Input: part model. Units: mm. Frame: model coordinates. A direction names the side the tool comes from. Give positions to 0.01 mm unless a question says otherwise; leave off trailing zeros. Loops run counter-clockwise (first coordinate to the right, second up) from the corner with the lowest first, then second, coordinate; pieces in that order, holes last. Notation, with made-up numbers: M 71.25,-22.5 L 102.25,-22.5 A20 ccw 102.25,-5.5 Z; hole C -21.5,46 d9. An arc over 180 degrees is marked long. Use CSV: the item, a comma, the result in double quotes. Start each with the question number.
Q1. Pin query (flat end, axial travel): pin 1 (20.5 mm diameter, centred on x = 49.5, z = 49.5, fed in from -Y); pin 2 (14.5 mm diameter, centred on x = -49.5, z = 49.5, fed in from -Y); pin 3 (7 mm diameter, centred on x = -45.96, z = 45.96, fed in from -Y). Return the tip coordinate at first contact, or that it passes through.
Q2. Section D-D, the plane y = -36. Output: boundary loops of the cut face in (x, z), plus the area to 3 significant figures.
Q3. Section C-C, the plane x = 69.5. Output: boundary loops of the cut face in (y, z).
Q4. Pull-direction query (X, two-part tool) for faces 6 (the cylindrical face through (-34.05, 53.52, -41.21)), 7 (the flat face through (88.5, -1, 1)), 8 (the flat face through (-21, 56.475, 29)); classes: released by +X, released by -X, zero draft, split by the parting line, or undercut.
Q5. Section A-A, the plane x = 0. Output: boundary loops of the cut face in (y, z), plus the area to 3 significant figures.
Q6. Section B-B, the plane z = 0. Output: boundary loops of the cut face in (x, y), plus the area to 3 significant figures.
Q7. Reachability of faces 1 (the flat face through (-0.413, -54.646, 92.014)), 2 (the flat face through (-41, -56.475, -40)), 3 (the cylindrical face through (52.945, -53.517, 57.811)), 4 (the flat face through (-19.5, 50.475, 29.4)), 5 (the cylindrical face through (-5.48, 53.52, -44.86)) from +Z, -Z, +X, -X, +Y, -Y: full face, straight path, thin tool, end or side. Return the list, or none.
Q8. Material intervals for line 1 along X through (y, z) = (22, 34); line 2 along Y through (x, z) = (65.5, -42); line 3 along Y through (x, z) = (-18, -38), sorted ascending.
from build123d import *

# Parameters (mm, degrees)
SKETCH1_W           = 177
SKETCH1_H           = 112.94900091
SKETCH1_W_2         = 165
SKETCH1_H_2         = 100.94900091
EXTRUDE_THIN1_DEPTH = 92.5
CUT_EXTRUDE1_REACH  = 172.722
SKETCH2_R           = 35
SKETCH2_R_2         = 6
SKETCH3_R           = 50
SKETCH3_R_2         = 9
CUT_EXTRUDE2_DEPTH  = 10
CUT_EXTRUDE3_DEPTH  = 208.544258417
CIRPATTERN1_COUNT   = 4
SKETCH5_R           = 9
CUT_EXTRUDE4_DEPTH  = 10


with BuildPart() as part:
    # Sketch1 → Extrude-Thin1 (new, symmetric)
    with BuildSketch(Plane.XY):
        Rectangle(SKETCH1_W, SKETCH1_H)
        Rectangle(SKETCH1_W_2, SKETCH1_H_2, mode=Mode.SUBTRACT)
    extrude(amount=EXTRUDE_THIN1_DEPTH, both=True)

    # Sketch2 → Cut-Extrude1 (cut, up to next)
    with BuildSketch(Plane(origin=(0, 56.474500455, 0), x_dir=(1, 0, 0), z_dir=(0, 1, 0)), mode=Mode.PRIVATE) as cut_extrude1_sk1:
        with Locations(Location((0, 0, 0), (0, 0, 270))):
            Circle(SKETCH2_R)
    cut_extrude1_tool1 = extrude(cut_extrude1_sk1.sketch, amount=-CUT_EXTRUDE1_REACH, mode=Mode.PRIVATE) & part.part
    # Sketch2 → Cut-Extrude1 (cut, up to next)
    with BuildSketch(Plane(origin=(0, 56.474500455, 0), x_dir=(1, 0, 0), z_dir=(0, 1, 0)), mode=Mode.PRIVATE) as cut_extrude1_sk2:
        with Locations(Location((-35.355339059, -35.355339059, 0), (0, 0, 270))):
            Circle(SKETCH2_R_2)
    cut_extrude1_tool2 = extrude(cut_extrude1_sk2.sketch, amount=-CUT_EXTRUDE1_REACH, mode=Mode.PRIVATE) & part.part
    # Sketch2 → Cut-Extrude1 (cut, up to next)
    with BuildSketch(Plane(origin=(0, 56.474500455, 0), x_dir=(1, 0, 0), z_dir=(0, 1, 0)), mode=Mode.PRIVATE) as cut_extrude1_sk3:
        with Locations(Location((-45.961940777, -45.961940777, 0), (0, 0, 270))):
            Circle(SKETCH2_R_2)
    cut_extrude1_tool3 = extrude(cut_extrude1_sk3.sketch, amount=-CUT_EXTRUDE1_REACH, mode=Mode.PRIVATE) & part.part
    cut_extrude1_1 = cut_extrude1_tool1.solids().sort_by_distance((0, 56.4745, 0))[0]
    add(cut_extrude1_1, mode=Mode.SUBTRACT)
    cut_extrude1_2 = cut_extrude1_tool2.solids().sort_by_distance((-35.355339, 56.4745, 35.355339))[0]
    add(cut_extrude1_2, mode=Mode.SUBTRACT)
    cut_extrude1_3 = cut_extrude1_tool3.solids().sort_by_distance((-45.961941, 56.4745, 45.961941))[0]
    add(cut_extrude1_3, mode=Mode.SUBTRACT)
    cut_extrude1 = cut_extrude1_1 + cut_extrude1_2 + cut_extrude1_3  # Cut-Extrude1 as one shape, for the pattern or mirror that repeats it

    # Sketch3 → Cut-Extrude2 (cut)
    with BuildSketch(Plane.XZ.offset(56.474500455)):
        with Locations(Location((0, 0, 0), (0, 0, 270))):
            Circle(SKETCH3_R)
        with Locations(Location((-49.497474683, -49.497474683, 0), (0, 0, 270))):
            Circle(SKETCH3_R_2)
    cut_extrude2 = extrude(amount=-CUT_EXTRUDE2_DEPTH, mode=Mode.SUBTRACT)

    # Sketch4 → Cut-Extrude3 (cut, through all)
    with BuildSketch(Plane.ZY.offset(88.5)):
        Polygon((-92.5, -56.474500455), (-62.5, 56.474500455), (-92.5, 56.474500455), align=None)
    cut_extrude3 = extrude(amount=-CUT_EXTRUDE3_DEPTH, mode=Mode.SUBTRACT)

    # Mirror1: Cut-Extrude3 across plane
    add(cut_extrude3.mirror(Plane.XY), mode=Mode.SUBTRACT)

    # CirPattern1: Cut-Extrude1, Cut-Extrude2 ×4 about axis
    cirpattern1_axis = Axis((0, 0, 0), (0, 1, 0))
    add([cut_extrude1.rotate(cirpattern1_axis, i * 360 / CIRPATTERN1_COUNT) for i in range(1, CIRPATTERN1_COUNT)], mode=Mode.SUBTRACT)
    add([cut_extrude2.rotate(cirpattern1_axis, i * 360 / CIRPATTERN1_COUNT) for i in range(1, CIRPATTERN1_COUNT)], mode=Mode.SUBTRACT)

    # Sketch5 → Cut-Extrude4 (cut)
    with BuildSketch(Plane(origin=(0, 56.474500455, 0), x_dir=(1, 0, 0), z_dir=(0, 1, 0))):
        with Locations(Location((0, -52, 0), (0, 0, 270))):
            Circle(SKETCH5_R)
    cut_extrude4 = extrude(amount=-CUT_EXTRUDE4_DEPTH, mode=Mode.SUBTRACT)

    # Mirror2: Cut-Extrude4 across plane
    add(cut_extrude4.mirror(Plane.XY), mode=Mode.SUBTRACT)


solid = part.part
A:
1,pin 1,"y = -56.47"
1,pin 2,"y = 50.47"
1,pin 3,"through"
2,outline,"M -88.5,-87.06 L -82.5,-87.06 L -82.5,87.06 L -88.5,87.06 Z; M 82.5,-87.06 L 88.5,-87.06 L 88.5,87.06 L 82.5,87.06 Z"
2,area,"2,090 mm^2"
3,outline,"M -56.47,-92.5 L -50.47,-90.91 L -50.47,90.91 L -56.47,92.5 Z; M 50.47,-64.09 L 56.47,-62.5 L 56.47,62.5 L 50.47,64.09 Z"
4,face 6,"undercut"
4,face 7,"released by +X"
4,face 8,"zero draft"
5,outline,"M -56.47,-92.5 L -50.47,-90.91 L -50.47,-50 L -56.47,-50 Z; M -56.47,50 L -50.47,50 L -50.47,90.91 L -56.47,92.5 Z; M 50.47,-64.09 L 56.47,-62.5 L 56.47,-61 L 50.47,-61 Z; M 50.47,-43 L 56.47,-43 L 56.47,-35 L 50.47,-35 Z; M 50.47,35 L 56.47,35 L 56.47,43 L 50.47,43 Z; M 50.47,61 L 56.47,61 L 56.47,62.5 L 50.47,64.09 Z"
5,area,"624 mm^2"
6,outline,"M -88.5,-56.47 L -50,-56.47 L -50,-50.47 L -82.5,-50.47 L -82.5,50.47 L -35,50.47 L -35,56.47 L -88.5,56.47 Z; M 35,50.47 L 82.5,50.47 L 82.5,-50.47 L 50,-50.47 L 50,-56.47 L 88.5,-56.47 L 88.5,56.47 L 35,56.47 Z"
6,area,"2,320 mm^2"
7,face 1,"+Z, +X, -X, +Y"
7,face 2,"+Z, -Z, +X, -X, -Y"
7,face 3,"-Y"
7,face 4,"+Z, -Z"
7,face 5,"+Y"
8,line 1,"-88.5 to -82.5, 82.5 to 88.5"
8,line 2,"-56.47 to -50.47, 50.47 to 56.47"
8,line 3,"50.47 to 56.47"
